Source: CAD feature listing. Evaluate the final solid. Frame: model axes, mm. Round coordinates to 2 decimals unless told otherwise and drop trailing zeros. Loops run counter-clockwise (first coordinate to the right, second up) from the corner with the lowest first, then second, coordinate; pieces in that order, holes last.
Item 1: Section query A-A on y = 89. Return loops of the section in (x, z) (3 decimals), then the cut area to 3 significant figures.
Item 2: Ray query, L1, parallel to Y at x = 43.5, z = 0.3; L2, parallel to X at y = 29, z = 2. Return the intervals inside material, ascending.
Item 3: Section query C-C on x = 249. Return loops of the section in (y, z) (3 decimals).
```python
from build123d import *

# Parameters (mm, degrees)
SKETCH1_W           = 393.7
SKETCH1_H           = 101.6
BOSS_EXTRUDE1_DEPTH = 3.175
SKETCH2_W           = 393.4968
SKETCH2_H           = 101.3968
BOSS_EXTRUDE2_DEPTH = 3.175


with BuildPart() as part:
    # Sketch1 → Boss-Extrude1 (new body)
    with BuildSketch(Plane.XY):
        Polygon((0, 0), (400.05, 0), (400.05, 0.0254), (406.4, 0.0254), (406.4, 0), (406.4, 117.36705), (406.4, 117.34165), (400.05, 117.34165), (400.05, 117.36705), (0, 117.36705), align=None)
        with Locations((203.2, 58.683525)):
            Rectangle(SKETCH1_W, SKETCH1_H, mode=Mode.SUBTRACT)
    extrude(amount=BOSS_EXTRUDE1_DEPTH)

    # Sketch2 → Boss-Extrude2 (add)
    with BuildSketch(Plane.XY.offset(3.175)):
        Polygon((400.1516, 117.46865), (-0.1016, 117.46865), (-0.1016, -0.1016), (400.1516, -0.1016), (400.1516, -0.0762), (406.5016, -0.0762), (406.5016, 117.44325), (400.1516, 117.44325), align=None)
        with Locations((203.2, 58.683525)):
            Rectangle(SKETCH2_W, SKETCH2_H, mode=Mode.SUBTRACT)
    extrude(amount=-BOSS_EXTRUDE2_DEPTH)


solid = part.part
```
Data:
1. outline: (-0.102, 0) - (6.452, 0) - (6.452, 3.175) - (-0.102, 3.175) - close; (399.948, 0) - (406.502, 0) - (406.502, 3.175) - (399.948, 3.175) - close
1. area: 41.6 mm2
2. L1: y = -0.1 to 7.99, 109.38 to 117.47
2. L2: x = -0.1 to 6.45, 399.95 to 406.5
3. outline: (-0.102, 0) - (7.985, 0) - (7.985, 3.175) - (-0.102, 3.175) - close; (109.382, 0) - (117.469, 0) - (117.469, 3.175) - (109.382, 3.175) - close
